from build123d import *

# Parameters (mm, degrees)
BOSS_EXTRUDE1_DEPTH      = 127
BOSS_EXTRUDE1_DEPTH_BACK = 19.547940452
BOSS_EXTRUDE3_DEPTH      = 31.75


with BuildPart() as part:
    # Sketch1 → Boss-Extrude1 (new, two sides)
    with BuildSketch(Plane.XY) as boss_extrude1_sk:
        Polygon((-38.1, 0), (38.1, 0), (33.02, 5.08), (-33.02, 5.08), align=None)
    extrude(amount=BOSS_EXTRUDE1_DEPTH)
    extrude(boss_extrude1_sk.sketch, amount=-BOSS_EXTRUDE1_DEPTH_BACK)

    # Sketch3 → Boss-Extrude3 (add, symmetric)
    with BuildSketch(Plane(origin=(0, 0, 0), x_dir=(0, 0, -1), z_dir=(1, 0, 0))):
        Polygon((0, 0), (9.75014649, 25.4), (4.67014649, 25.4), (-5.08, 0), align=None)
    extrude(amount=BOSS_EXTRUDE3_DEPTH, both=True)

    # SurfaceCut2
    split(bisect_by=Plane(origin=(0, 0, 0), x_dir=(-1, 0, 0), z_dir=(0, -0.3583679495453043, -0.9335804264972002)), keep=Keep.BOTTOM)


solid = part.part
Input: part model. Units: mm. Frame: model coordinates. A direction names the side the tool comes from. Coordinates: 2 decimals unless noted, no trailing zeros. Order: outer loops, then holes, each group sorted by start corner. A loop starts at its lowest first (then second) coordinate and runs counter-clockwise, first axis right, second up.
1. Ray query, line 1 along Y through (x, z) = (32, 15.5); line 2 along Z through (x, y) = (23, 6.75); line 3 along Z through (x, y) = (-20.5, 8). Return the intervals inside material, ascending.
Checked values:
line 1: y = 0 to 5.08
line 2: z = -2.59 to 2.49
line 3: z = -3.07 to 2.01
2. Cut plane A-A, the plane x = -9.5. Return loops of the section in (y, z), plus the area to 3 significant figures.
Checked values:
outline: (0, 0) - (25.4, -9.75) - (25.4, -4.67) - (5.08, 3.13) - (5.08, 127) - (0, 127) - close
area: 753 mm2
3. Access query for faces 1 (the flat face through (-1, 3, 127)), 2 (the flat face through (-31.75, 15, -3)), 3 (the flat face through (31.75, 15, -3)). Directions: +Z, -Z, +X, -X, +Y, -Y. A direction counts if a zero-diameter tool reaches every point of the face in a straight line with its end or side. Return the directions, or none.
Checked values:
face 1: +Z, +X, -X, +Y, -Y
face 2: +Z, -Z, -X, +Y
face 3: +Z, -Z, +X, +Y
4. Cut plane C-C, the plane y = 3.25. Return loops of the section in (x, z).
Checked values:
outline: (-34.85, -1.25) - (34.85, -1.25) - (34.85, 127) - (-34.85, 127) - close
5. Cut plane B-B, the plane z = 20. Return loops of the section in (x, y).
Checked values:
outline: (-38.1, 0) - (38.1, 0) - (33.02, 5.08) - (-33.02, 5.08) - close
6. Contact query for flat-ended pins moving along their axis: P1, Ø6, axis at y = 5, z = 12.5, coming from the -X side; P2, Ø6, axis at x = 8.5, y = 15.5, coming from the -Z side; P3, Ø5, axis at x = -13, z = 106, coming from the +Y side. Output: stop coordinate, or through.
Checked values:
P1: stops at x = -36.1
P2: stops at z = -7.1
P3: stops at y = 5.08
